from build123d import *

# Parameters (mm, degrees)
SALIENTE_EXTRUIR1_DEPTH      = 80
SALIENTE_EXTRUIR1_DEPTH_BACK = 80
CROQUIS2_W                   = 35
CROQUIS2_H                   = 50
CORTAR_EXTRUIR1_DEPTH        = 3
CROQUIS3_R                   = 2.5
CROQUIS3_R_2                 = 5
CORTAR_EXTRUIR2_DEPTH        = 3
SALIENTE_EXTRUIR2_DEPTH      = 3
CROQUIS5_R                   = 16
CORTAR_EXTRUIR3_DEPTH        = 3


with BuildPart() as part:
    # Croquis1 → Saliente-Extruir1 (new body, two sides)
    with BuildSketch(Plane.XY) as saliente_extruir1_sk:
        Polygon((0, 0), (0, 38), (3, 38), (3, 3), (38, 3), (38, 0), align=None)
    extrude(amount=SALIENTE_EXTRUIR1_DEPTH)
    extrude(saliente_extruir1_sk.sketch, amount=-SALIENTE_EXTRUIR1_DEPTH_BACK)

    # Croquis2 → Cortar-Extruir1 (cut)
    with BuildSketch(Plane(origin=(0, 3, 0), x_dir=(1, 0, 0), z_dir=(0, 1, 0))):
        with Locations((20.5, 0)):
            Rectangle(CROQUIS2_W, CROQUIS2_H)
    extrude(amount=-CORTAR_EXTRUIR1_DEPTH, mode=Mode.SUBTRACT)

    # Croquis3 → Cortar-Extruir2 (cut)
    with BuildSketch(Plane.ZY):
        with Locations((71.5, 22)):
            Circle(CROQUIS3_R)
        with Locations((55, 22)):
            Circle(CROQUIS3_R_2)
        with Locations((38.5, 22)):
            Circle(CROQUIS3_R)
        with Locations((-38.5, 22)):
            Circle(CROQUIS3_R)
        with Locations((-55, 22)):
            Circle(CROQUIS3_R_2)
        with Locations((-71.5, 22)):
            Circle(CROQUIS3_R)
    extrude(amount=-CORTAR_EXTRUIR2_DEPTH, mode=Mode.SUBTRACT)

    # Croquis4 → Saliente-Extruir2 (add)
    with BuildSketch(Plane.ZY):
        Polygon((27.5, 38), (17.5, 48), (-17.5, 48), (-27.5, 38), align=None)
    extrude(amount=-SALIENTE_EXTRUIR2_DEPTH)

    # Croquis5 → Cortar-Extruir3 (cut)
    with BuildSketch(Plane.ZY):
        with Locations((0, 22)):
            Circle(CROQUIS5_R)
    extrude(amount=-CORTAR_EXTRUIR3_DEPTH, mode=Mode.SUBTRACT)


solid = part.part
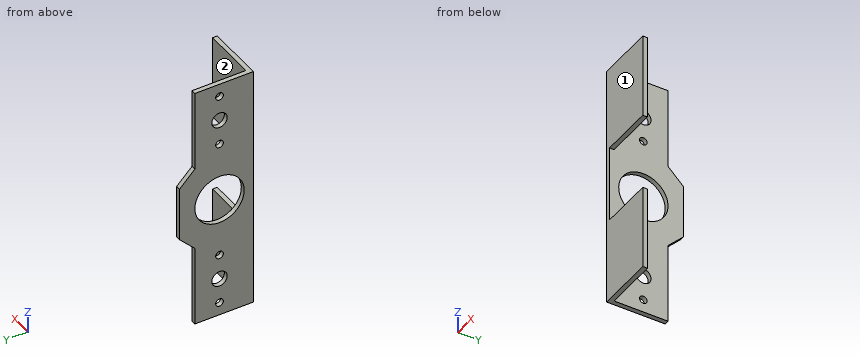
Work out the finished part from the listing and answer in its coordinate system (mm). Face numbers are marked on the shaded views. A direction names the side the tool comes from. Give positions to 0.01 mm unless a question says otherwise; leave off trailing zeros. Loops run counter-clockwise (first coordinate to the right, second up) from the corner with the lowest first, then second, coordinate; pieces in that order, holes last. Notation, with made-up numbers: (-39, 75) - (-8, 75) arc R30 ccw to (-8, 103) - close; hole circle Ø7 at (-16.5, 51). An arc over 180 degrees is marked (long way). Answer in a Markdown table with one row per item.
(1) A tool of negligible diameter and unlimited length cuts with its end or side. For the marked faces 1 and 2, from which of +Z, -Z, +X, -X, +Y, -Y can it reach the whole face along a straight path? Write none if from no direction.
Results list:
| item | result |
|---|---|
| face 1 | +Z, -Z, +X, -X, -Y |
| face 2 | +Z, -Z, +X, +Y |
(2) Section C-C (y = 33) is taken. Give the vertices of the cut face in (x, z).
Results list:
| item | result |
|---|---|
| outline | (0, -80) - (3, -80) - (3, -11.62) - (0, -11.62) - close; (0, 11.62) - (3, 11.62) - (3, 80) - (0, 80) - close |
(3) Section A-A (z = 55) is taken. Give the vertices of the cut face in (x, y), and give its area (3 significant figures).
Results list:
| item | result |
|---|---|
| outline | (0, 0) - (38, 0) - (38, 3) - (3, 3) - (3, 17) - (0, 17) - close; (0, 27) - (3, 27) - (3, 38) - (0, 38) - close |
| area | 189 mm² |
(4) Section D-D (z = -71.5) is taken. Give the vertices of the cut face in (x, y).
Results list:
| item | result |
|---|---|
| outline | (0, 0) - (38, 0) - (38, 3) - (3, 3) - (3, 19.5) - (0, 19.5) - close; (0, 24.5) - (3, 24.5) - (3, 38) - (0, 38) - close |
(5) Flat-ended cylindrical pins translate along their axes: pin 1 Ø8 at (y, z) = (22, -71.5) entering from +X; pin 2 Ø2.5 at (x, z) = (2, -55.5) entering from +Y; pin 3 Ø10.5 at (x, z) = (14, -49.5) entering from +Y. Find the tip coordinate at first contact, or state that the pin passes through.
Results list:
| item | result |
|---|---|
| pin 1 | stops at x = 3 |
| pin 2 | stops at y = 38 |
| pin 3 | stops at y = 3 |
(6) Consider L1, parallel to Y at x = 2.05, z = -38.5; L2, parallel to Y at x = 0.8, z = -55; L3, parallel to X at y = 32.5, z = 13. Determine where each line is inside the solid, lowest interval first. Write a range as [from, to].
Results list:
| item | result |
|---|---|
| L1 | y = [0, 19.5], [24.5, 38] |
| L2 | y = [0, 17], [27, 38] |
| L3 | x = [0, 3] |
(7) Section B-B (x = 7) is taken. Give the vertices of the cut face in (y, z).
Results list:
| item | result |
|---|---|
| outline | (0, -80) - (3, -80) - (3, -25) - (0, -25) - close; (0, 25) - (3, 25) - (3, 80) - (0, 80) - close |
